Part model, mm, in its own coordinate system. A direction names the side the tool comes from. Give positions to 0.01 mm unless a question says otherwise; leave off trailing zeros. Order: outer loops, then holes, each group sorted by start corner. A loop starts at its lowest first (then second) coordinate and runs counter-clockwise, first axis right, second up. Notation, with made-up numbers: M 34.5,-1.75 L 75.5,-1.75 A8 cw 75.5,7.25 Z; hole C 41.5,88 d7. An arc over 180 degrees is marked long. Return JSON: item names as keys, results as strings.
from build123d import *

# Parameters (mm, degrees)
F0_R     = 6.65
F0_R_2   = 2.55
F1_DEPTH = 1.2
F2_DEPTH = 8
F3_R     = 0.3


# Not quite as in the source:
# - a feature names something its author has since deleted; it is built from what else it names


with BuildPart() as f1:
    # F0 (on Top) → F1 (new body)
    with BuildSketch(Plane.XY):
        with BuildLine():
            Line((9.6529388756, 1.998378199), (20.2717385681, 1.998378199))
            ThreePointArc((20.2717385681, 1.998378199), (14.4037651328, 14.4037651328), (1.998378199, 20.2717385681))
            Line((1.998378199, 20.2717385681), (1.998378199, 9.6529388756))
            ThreePointArc((1.998378199, 9.6529388756), (2.3354389744, 8.5417984096), (3.2330113343, 7.8051798106))
            ThreePointArc((3.2330113343, 7.8051798106), (5.9738260003, 5.9738260003), (7.8051798106, 3.2330113343))
            ThreePointArc((7.8051798106, 3.2330113343), (8.5417984096, 2.3354389744), (9.6529388756, 1.998378199))
        make_face()
        with BuildLine():
            Line((-1.998378199, 9.6529388756), (-1.998378199, 20.2717385681))
            ThreePointArc((-1.998378199, 20.2717385681), (-14.4037651328, 14.4037651328), (-20.2717385681, 1.998378199))
            Line((-20.2717385681, 1.998378199), (-9.6529388756, 1.998378199))
            ThreePointArc((-9.6529388756, 1.998378199), (-8.5417984096, 2.3354389744), (-7.8051798106, 3.2330113343))
            ThreePointArc((-7.8051798106, 3.2330113343), (-5.9738260003, 5.9738260003), (-3.2330113343, 7.8051798106))
            ThreePointArc((-3.2330113343, 7.8051798106), (-2.3354389744, 8.5417984096), (-1.998378199, 9.6529388756))
        make_face()
        with BuildLine():
            ThreePointArc((-20.2717385681, -1.998378199), (-14.4037651328, -14.4037651328), (-1.998378199, -20.2717385681))
            Line((-1.998378199, -20.2717385681), (-1.998378199, -9.6529388756))
            ThreePointArc((-1.998378199, -9.6529388756), (-2.3354389744, -8.5417984096), (-3.2330113343, -7.8051798106))
            ThreePointArc((-3.2330113343, -7.8051798106), (-5.9738260003, -5.9738260003), (-7.8051798106, -3.2330113343))
            ThreePointArc((-7.8051798106, -3.2330113343), (-8.5417984096, -2.3354389744), (-9.6529388756, -1.998378199))
            Line((-9.6529388756, -1.998378199), (-20.2717385681, -1.998378199))
        make_face()
        with BuildLine():
            ThreePointArc((1.998378199, -20.2717385681), (14.4037651328, -14.4037651328), (20.2717385681, -1.998378199))
            Line((20.2717385681, -1.998378199), (9.6529388756, -1.998378199))
            ThreePointArc((9.6529388756, -1.998378199), (8.5417984096, -2.3354389744), (7.8051798106, -3.2330113343))
            ThreePointArc((7.8051798106, -3.2330113343), (5.9738260003, -5.9738260003), (3.2330113343, -7.8051798106))
            ThreePointArc((3.2330113343, -7.8051798106), (2.3354389744, -8.5417984096), (1.998378199, -9.6529388756))
            Line((1.998378199, -9.6529388756), (1.998378199, -20.2717385681))
        make_face()
        with BuildLine():
            ThreePointArc((20.2717385681, -1.998378199), (20.3454198117, -1.0003962634), (20.37, 0))
            ThreePointArc((20.37, 0), (20.3454198117, 1.0003962634), (20.2717385681, 1.998378199))
            Line((20.2717385681, 1.998378199), (9.6529388756, 1.998378199))
            ThreePointArc((9.6529388756, 1.998378199), (8.5417984096, 2.3354389744), (7.8051798106, 3.2330113343))
            ThreePointArc((7.8051798106, 3.2330113343), (5.9738260003, 5.9738260003), (3.2330113343, 7.8051798106))
            ThreePointArc((3.2330113343, 7.8051798106), (2.3354389744, 8.5417984096), (1.998378199, 9.6529388756))
            Line((1.998378199, 9.6529388756), (1.998378199, 20.2717385681))
            ThreePointArc((1.998378199, 20.2717385681), (0, 20.37), (-1.998378199, 20.2717385681))
            Line((-1.998378199, 20.2717385681), (-1.998378199, 9.6529388756))
            ThreePointArc((-1.998378199, 9.6529388756), (-2.3354389744, 8.5417984096), (-3.2330113343, 7.8051798106))
            ThreePointArc((-3.2330113343, 7.8051798106), (-5.9738260003, 5.9738260003), (-7.8051798106, 3.2330113343))
            ThreePointArc((-7.8051798106, 3.2330113343), (-8.5417984096, 2.3354389744), (-9.6529388756, 1.998378199))
            Line((-9.6529388756, 1.998378199), (-20.2717385681, 1.998378199))
            ThreePointArc((-20.2717385681, 1.998378199), (-20.37, 0), (-20.2717385681, -1.998378199))
            Line((-20.2717385681, -1.998378199), (-9.6529388756, -1.998378199))
            ThreePointArc((-9.6529388756, -1.998378199), (-8.5417984096, -2.3354389744), (-7.8051798106, -3.2330113343))
            ThreePointArc((-7.8051798106, -3.2330113343), (-5.9738260003, -5.9738260003), (-3.2330113343, -7.8051798106))
            ThreePointArc((-3.2330113343, -7.8051798106), (-2.3354389744, -8.5417984096), (-1.998378199, -9.6529388756))
            Line((-1.998378199, -9.6529388756), (-1.998378199, -20.2717385681))
            ThreePointArc((-1.998378199, -20.2717385681), (0, -20.37), (1.998378199, -20.2717385681))
            Line((1.998378199, -20.2717385681), (1.998378199, -9.6529388756))
            ThreePointArc((1.998378199, -9.6529388756), (2.3354389744, -8.5417984096), (3.2330113343, -7.8051798106))
            ThreePointArc((3.2330113343, -7.8051798106), (5.9738260003, -5.9738260003), (7.8051798106, -3.2330113343))
            ThreePointArc((7.8051798106, -3.2330113343), (8.5417984096, -2.3354389744), (9.6529388756, -1.998378199))
            Line((9.6529388756, -1.998378199), (20.2717385681, -1.998378199))
        make_face()
        Circle(F0_R, mode=Mode.SUBTRACT)
        Circle(F0_R)
        Circle(F0_R_2, mode=Mode.SUBTRACT)
    extrude(amount=-F1_DEPTH)

    # F0 (on Top) → F2 (join)
    with BuildSketch(Plane.XY):
        with BuildLine():
            ThreePointArc((20.2717385681, -1.998378199), (20.3454198117, -1.0003962634), (20.37, 0))
            ThreePointArc((20.37, 0), (20.3454198117, 1.0003962634), (20.2717385681, 1.998378199))
            Line((20.2717385681, 1.998378199), (9.6529388756, 1.998378199))
            ThreePointArc((9.6529388756, 1.998378199), (8.5417984096, 2.3354389744), (7.8051798106, 3.2330113343))
            ThreePointArc((7.8051798106, 3.2330113343), (5.9738260003, 5.9738260003), (3.2330113343, 7.8051798106))
            ThreePointArc((3.2330113343, 7.8051798106), (2.3354389744, 8.5417984096), (1.998378199, 9.6529388756))
            Line((1.998378199, 9.6529388756), (1.998378199, 20.2717385681))
            ThreePointArc((1.998378199, 20.2717385681), (0, 20.37), (-1.998378199, 20.2717385681))
            Line((-1.998378199, 20.2717385681), (-1.998378199, 9.6529388756))
            ThreePointArc((-1.998378199, 9.6529388756), (-2.3354389744, 8.5417984096), (-3.2330113343, 7.8051798106))
            ThreePointArc((-3.2330113343, 7.8051798106), (-5.9738260003, 5.9738260003), (-7.8051798106, 3.2330113343))
            ThreePointArc((-7.8051798106, 3.2330113343), (-8.5417984096, 2.3354389744), (-9.6529388756, 1.998378199))
            Line((-9.6529388756, 1.998378199), (-20.2717385681, 1.998378199))
            ThreePointArc((-20.2717385681, 1.998378199), (-20.37, 0), (-20.2717385681, -1.998378199))
            Line((-20.2717385681, -1.998378199), (-9.6529388756, -1.998378199))
            ThreePointArc((-9.6529388756, -1.998378199), (-8.5417984096, -2.3354389744), (-7.8051798106, -3.2330113343))
            ThreePointArc((-7.8051798106, -3.2330113343), (-5.9738260003, -5.9738260003), (-3.2330113343, -7.8051798106))
            ThreePointArc((-3.2330113343, -7.8051798106), (-2.3354389744, -8.5417984096), (-1.998378199, -9.6529388756))
            Line((-1.998378199, -9.6529388756), (-1.998378199, -20.2717385681))
            ThreePointArc((-1.998378199, -20.2717385681), (0, -20.37), (1.998378199, -20.2717385681))
            Line((1.998378199, -20.2717385681), (1.998378199, -9.6529388756))
            ThreePointArc((1.998378199, -9.6529388756), (2.3354389744, -8.5417984096), (3.2330113343, -7.8051798106))
            ThreePointArc((3.2330113343, -7.8051798106), (5.9738260003, -5.9738260003), (7.8051798106, -3.2330113343))
            ThreePointArc((7.8051798106, -3.2330113343), (8.5417984096, -2.3354389744), (9.6529388756, -1.998378199))
            Line((9.6529388756, -1.998378199), (20.2717385681, -1.998378199))
        make_face()
        Circle(F0_R, mode=Mode.SUBTRACT)
    extrude(amount=F2_DEPTH)

    # F3
    f3_edges = [f1.edges().sort_by_distance(p)[0] for p in [
        (-1.998378, -20.271739, -1.2),
    ]]
    fillet(f3_edges, radius=F3_R)


solid = f1.part
Q1. Probe line 1 along Y through (x, z) = (0, -0.55); line 2 along Y through (x, z) = (0, 3.25); line 3 along Z through (x, y) = (3, 1.5). List the from-to ranges inside material, lowest first.
Established:
{"line 1": "y = -20.37 to -2.55, 2.55 to 20.37", "line 2": "y = -20.37 to -6.65, 6.65 to 20.37", "line 3": "z = -1.2 to 0"}
Q2. Band-saw the part on B-B (z = 2). Give the cut face in (x, y).
Established:
{"outline": "M -20.27,-2 L -9.65,-2 A2 cw -7.81,-3.23 A8.45 ccw -3.23,-7.81 A2 cw -2,-9.65 L -2,-20.27 A20.37 ccw 2,-20.27 L 2,-9.65 A2 cw 3.23,-7.81 A8.45 ccw 7.81,-3.23 A2 cw 9.65,-2 L 20.27,-2 A20.37 ccw 20.27,2 L 9.65,2 A2 cw 7.81,3.23 A8.45 ccw 3.23,7.81 A2 cw 2,9.65 L 2,20.27 A20.37 ccw -2,20.27 L -2,9.65 A2 cw -3.23,7.81 A8.45 ccw -7.81,3.23 A2 cw -9.65,2 L -20.27,2 A20.37 ccw Z; hole C 0,0 d13.3"}
Q3. Two-plate mould, pull along Y, no slides. Class faces 5 (the cylindrical face through (5.94, -6.01, 3.94)), 6 (the flat face through (3, 0, 0)), 7 (the flat face through (-1.998, -15, 4)): +Y half, -Y half, draft (parallel to the pull), parting line (faces both ways), or undercut.
Established:
{"face 5": "-Y half", "face 6": "undercut", "face 7": "draft"}
Q4. Band-saw the part on A-A (x = 0). Give the cut face in (y, z).
Established:
{"outline": "M -20.37,-0.9 A0.3 ccw -20.07,-1.2 L -2.55,-1.2 L -2.55,0 L -6.65,0 L -6.65,8 L -20.37,8 Z; M 2.55,-1.2 L 20.07,-1.2 A0.3 ccw 20.37,-0.9 L 20.37,8 L 6.65,8 L 6.65,0 L 2.55,0 Z"}
Q5. Pin check, flat tips, straight feed: pin 1 (5.5 mm diameter, centred on x = -13.5, y = 15, fed in from +Z); pin 2 (1 mm diameter, centred on x = -15, z = 6, fed in from +Y); pin 3 (3 mm diameter, centred on y = 6, z = 2, fed in from -X). Stop position of each tip, or through.
Established:
{"pin 1": "stops at z = 0", "pin 2": "stops at y = 2", "pin 3": "stops at x = -7.15"}
Q6. 3-axis set-ups, long thin cutter, end or side, ignore diameter. For faces 1 (the cylindrical face through (2.3, -8.6, 3.9)), 2 (the flat face through (15, 1.998, 4)), 3 (the cylindrical face through (-2.345, -8.528, 3.944)), 4 (the flat face through (-9, 9, 0)): which of +Z, -Z, +X, -X, +Y, -Y reach the whole face in a straight line?
Established:
{"face 1": "+Z, +X, -Y", "face 2": "+Z, +X, +Y", "face 3": "+Z, -X, -Y", "face 4": "+Z, -X, +Y"}
